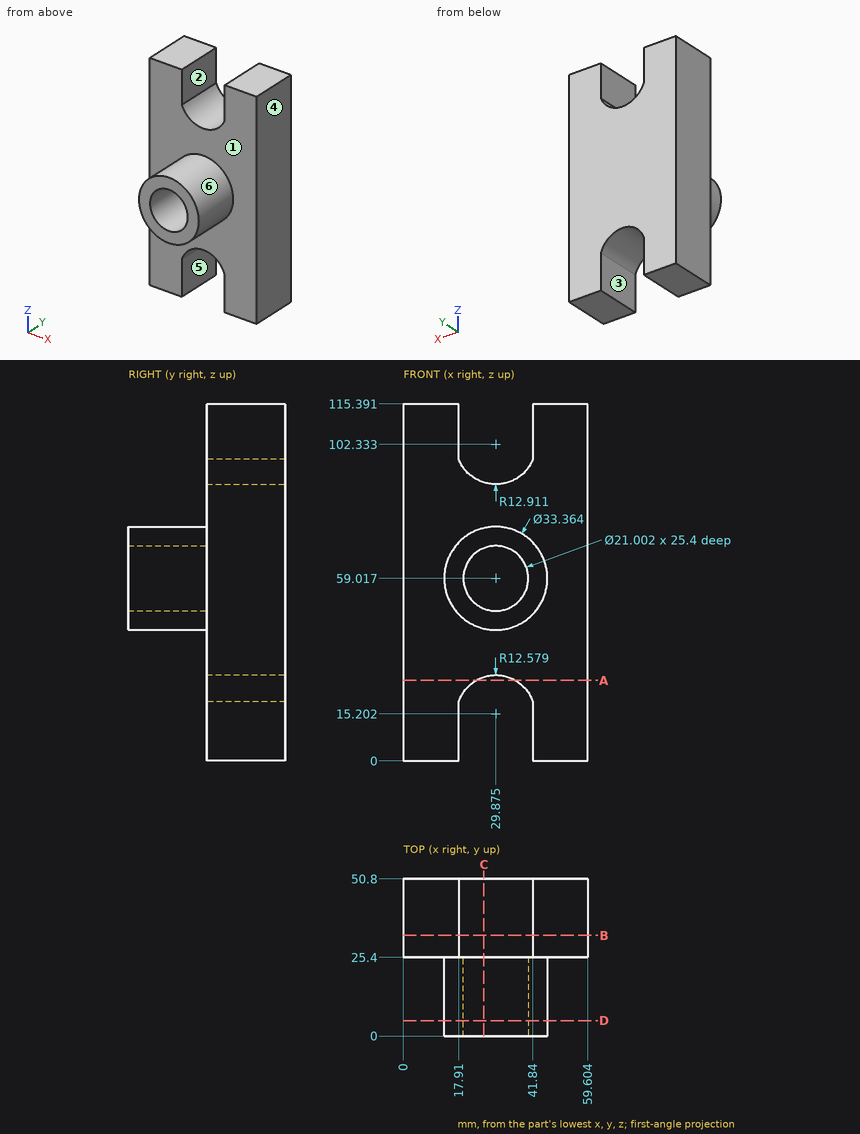
Can you work these out from the drawing? Everything is in mm from the part's minimum corner. A direction names the side the tool comes from. Give positions to 0.01 mm unless a question says otherwise; leave off trailing zeros. Loops run counter-clockwise (first coordinate to the right, second up) from the corner with the lowest first, then second, coordinate; pieces in that order, holes last. Notation, with made-up numbers: (-37, 9) -> (-7, 9) arc R27 cw to (-7, 43) -> close; hole circle Ø3 at (72, 25.25). An arc over 180 degrees is marked (long way). Return JSON: item names as keys, results as strings.
Item 1: If we section it at D-D on y = 5: List the corners of the cut face in (x, z) for me (1 decimal), plus the area to 3 significant figures.
Geometry results:
{"outline": "circle Ø33.4 at (29.9, 59); hole circle Ø21 at (29.9, 59)", "area": "528 mm²"}
Item 2: If we section it at A-A on z = 26: List the corners of the cut face in (x, y) for me.
Geometry results:
{"outline": "(0, 25.4) -> (23.42, 25.4) -> (23.42, 50.8) -> (0, 50.8) -> close; (36.33, 25.4) -> (59.6, 25.4) -> (59.6, 50.8) -> (36.33, 50.8) -> close"}
Item 3: I'm going to push a flat-ended pin straight in: pin 1 (1.5 mm diameter, centred on x = 36.5, z = 63, fed in from -Y). Where does the tip first touch, or does it pass through?
Geometry results:
{"pin 1": "stops at y = 25.4"}
Item 4: I need wall thicknesses on L1, parallel to X at y = 46, z = 104.5; L2, parallel to Y at x = 25.5, z = 53; L3, parallel to X at y = 34.5, z = 22 (1 decimal). Which ranges of each line are inside material? Lowest first, please. Write a range as from..to.
Geometry results:
{"L1": "x = 0..17.91, 41.84..59.6", "L2": "y = 25.4..50.8", "L3": "x = 0..19.3, 40.5..59.6"}
Item 5: If we section it at B-B on y = 32.5: List the corners of the cut face in (x, z) for me (1 decimal), plus the area to 3 significant figures.
Geometry results:
{"outline": "(0, 0) -> (17.9, 0) -> (17.9, 19.1) arc R12.6 cw to (41.8, 19.1) -> (41.8, 0) -> (59.6, 0) -> (59.6, 115.4) -> (41.8, 115.4) -> (41.8, 97.5) arc R12.9 cw to (17.9, 97.5) -> (17.9, 115.4) -> (0, 115.4) -> close", "area": "5,700 mm²"}
Item 6: Which directions (+Z, -Z, +X, -X, +Y, -Y) give clear straight access to the entire face, cutting with the end or side of a thin tool? Please do the marked faces 1, 2 and 3.
Geometry results:
{"face 1": "-Y", "face 2": "+Z, +Y, -Y", "face 3": "-Z, +Y, -Y"}
Item 7: If we section it at C-C on x = 26: List the corners of the cut face in (y, z) for me, plus the area to 4 significant figures.
Geometry results:
{"outline": "(0, 42.79) -> (25.4, 42.79) -> (25.4, 27.17) -> (50.8, 27.17) -> (50.8, 90.02) -> (25.4, 90.02) -> (25.4, 75.24) -> (0, 75.24) -> (0, 68.78) -> (25.4, 68.78) -> (25.4, 49.26) -> (0, 49.26) -> close", "area": "1,925 mm²"}
Item 8: We'd pull the mould along X, two halves only. Please class the marked faces 4, 5 and 6: +X half, -X half, draft (parallel to the pull), parting line (faces both ways), or undercut.
Geometry results:
{"face 4": "+X half", "face 5": "undercut", "face 6": "parting line"}
